from build123d import *

# Parameters (mm, degrees)
SKETCH1_R             = 115
BOSS_EXTRUDE1_DEPTH   = 6.4
CUT_EXTRUDE1_DEPTH    = 7.5
SKETCH3_R             = 1.75
CUT_EXTRUDE2_DEPTH    = 7.4
SKETCH4_R             = 2
CUT_EXTRUDE3_DEPTH    = 7.4
SKETCH5_R             = 3
CUT_EXTRUDE4_DEPTH    = 7.4
F_3_0MM_DOWEL_HOLE1_D = 3


with BuildPart() as part:
    # Sketch1 → Boss-Extrude1 (new body)
    with BuildSketch(Plane(origin=(0, 0, 0), x_dir=(1, 0, 0), z_dir=(0, 1, 0))):
        Circle(SKETCH1_R)
    extrude(amount=BOSS_EXTRUDE1_DEPTH)

    # Sketch2 → Cut-Extrude1 (cut)
    with BuildSketch(Plane(origin=(0, 6.4, 0), x_dir=(1, 0, 0), z_dir=(0, 1, 0))):
        with BuildLine():
            Line((-105.830052443, 45), (-70.830052443, 45))
            Line((-70.830052443, 45), (-70.830052443, -45))
            Line((-70.830052443, -45), (-105.830052443, -45))
            ThreePointArc((-105.830052443, -45), (-115, 0), (-105.830052443, 45))
        make_face()
        with BuildLine():
            Line((105.830052443, -45), (70.830052443, -45))
            Line((70.830052443, -45), (70.830052443, 45))
            Line((70.830052443, 45), (105.830052443, 45))
            ThreePointArc((105.830052443, 45), (115, 0), (105.830052443, -45))
        make_face()
    extrude(amount=-CUT_EXTRUDE1_DEPTH, mode=Mode.SUBTRACT)

    # Sketch3 → Cut-Extrude2 (cut, through all)
    with BuildSketch(Plane(origin=(0, 6.4, 0), x_dir=(1, 0, 0), z_dir=(0, 1, 0))):
        with Locations((-66.830052443, 0.75)):
            Circle(SKETCH3_R)
        with Locations((-66.830052443, -14.75)):
            Circle(SKETCH3_R)
        with Locations((66.830052443, -0.75)):
            Circle(SKETCH3_R)
        with Locations((66.830052443, 14.75)):
            Circle(SKETCH3_R)
    extrude(amount=-CUT_EXTRUDE2_DEPTH, mode=Mode.SUBTRACT)

    # Sketch4 → Cut-Extrude3 (cut, through all)
    with BuildSketch(Plane(origin=(0, 6.4, 0), x_dir=(1, 0, 0), z_dir=(0, 1, 0))):
        with Locations((30.525, 36.93)):
            Circle(SKETCH4_R)
        with Locations((-30.525, 36.93)):
            Circle(SKETCH4_R)
        with Locations((-30.525, 73.07)):
            Circle(SKETCH4_R)
    extrude(amount=-CUT_EXTRUDE3_DEPTH, mode=Mode.SUBTRACT)

    # Sketch5 → Cut-Extrude4 (cut, through all)
    with BuildSketch(Plane(origin=(0, 6.4, 0), x_dir=(1, 0, 0), z_dir=(0, 1, 0))):
        with Locations((-40, -30)):
            Circle(SKETCH5_R)
        with Locations((40, -30)):
            Circle(SKETCH5_R)
        with Locations((40, -70)):
            Circle(SKETCH5_R)
        with Locations((-40, -70)):
            Circle(SKETCH5_R)
    extrude(amount=-CUT_EXTRUDE4_DEPTH, mode=Mode.SUBTRACT)

    # Ø3.0mm Dowel Hole1 (through all)
    with Locations(Plane(origin=(0, 0, 0), x_dir=(-1, 0, 0), z_dir=(0, -1, 0))):
        with Locations((-55, 65), (55, 65), (55, -65), (-55, -65)):
            Hole(F_3_0MM_DOWEL_HOLE1_D / 2)


solid = part.part
Source: CAD feature listing. Evaluate the final solid. Frame: model axes, mm. A direction names the side the tool comes from. Give positions to 0.01 mm unless a question says otherwise; leave off trailing zeros. Loops run counter-clockwise (first coordinate to the right, second up) from the corner with the lowest first, then second, coordinate; pieces in that order, holes last. Notation, with made-up numbers: (14.25, -32.5) -> (51.25, -32.5) arc R17 ccw to (51.25, -1.5) -> close; hole circle Ø8 at (56, 69.25). An arc over 180 degrees is marked (long way). Use a Markdown table: item, result. Add a question column.
1) Section query A-A, the plane y = 2.75. Count the separate pieces of the cut face and the enclosed holes in it, then the cut area to 3 significant figures.
2) Line query: line 1 along X through (y, z) = (3.25, -36.93) (3 decimals); line 2 along X through (y, z) = (4.25, 30); line 3 along Z through (x, y) = (-40, 3.75). Output: solid intervals per line, ascending. Write a range as [from, to].
3) Reachability of faces 5 (the face through (-1.882, 3.155, 114.985)), 6 (the face through (89, 3, 45)), 7 (the face through (-88, 3, 45)) from +Z, -Z, +X, -X, +Y, -Y: full face, straight path, thin tool, end or side. Return the list, or none.
4) Pull-direction query (X, two-part tool) for faces 1 (the face through (-42.4, 3.2, 71.8)), 2 (the face through (37.6, 3.2, 71.8)), 3 (the face through (70.83, 3, 1)), 4 (the face through (88, 3, -45)); classes: +X half, -X half, draft (parallel to the pull), parting line (faces both ways), or undercut.
5) Section query D-D, the plane z = 82.5. Return the cut outline in (x, y).
6) Section query C-C, the plane x = 87. Return the cut outline in (y, z), then the cut area to 3 significant figures.
7) First-contact query: pin 1 (1.9 mm diameter, centred on x = -92, y = 3.5, fed in from +Z); pin 2 (1.5 mm diameter, centred on x = -78.5, y = 5, fed in from -Z). Flat tips, straight axial feed; report the tip coordinate or a pass-through.
8) Section query B-B, the plane x = 40. Return the cut outline in (y, z).
Numbers:
| question | item | result |
|---|---|---|
| 1 | separate pieces | 1 |
| 1 | enclosed holes | 15 |
| 1 | area | 33,900 mm2 |
| 2 | line 1 | x = [-70.83, -32.525], [-28.525, 28.525], [32.525, 70.83] |
| 2 | line 2 | x = [-70.83, -43], [-37, 37], [43, 70.83] |
| 2 | line 3 | z = [-107.82, 27], [33, 67], [73, 107.82] |
| 3 | face 5 | +Z, +Y, -Y |
| 3 | face 6 | +X, +Y, -Y |
| 3 | face 7 | -X, +Y, -Y |
| 4 | face 1 | undercut |
| 4 | face 2 | undercut |
| 4 | face 3 | +X half |
| 4 | face 4 | draft |
| 5 | outline | (-80.12, 0) -> (80.12, 0) -> (80.12, 6.4) -> (-80.12, 6.4) -> close |
| 6 | outline | (0, -75.21) -> (6.4, -75.21) -> (6.4, -45) -> (0, -45) -> close; (0, 45) -> (6.4, 45) -> (6.4, 75.21) -> (0, 75.21) -> close |
| 6 | area | 387 mm2 |
| 7 | pin 1 | stops at z = 70.25 |
| 7 | pin 2 | stops at z = -84.73 |
| 8 | outline | (0, -107.82) -> (6.4, -107.82) -> (6.4, 27) -> (0, 27) -> close; (0, 33) -> (6.4, 33) -> (6.4, 67) -> (0, 67) -> close; (0, 73) -> (6.4, 73) -> (6.4, 107.82) -> (0, 107.82) -> close |
